from build123d import *

# Parameters (mm, degrees)
SKETCH1_R           = 5
BOSS_EXTRUDE1_DEPTH = 2
BOSS_EXTRUDE2_DEPTH = 65.921828
FILLET1_R           = 12
FILLET2_R           = 12


with BuildPart() as part:
    # Sketch1 → Boss-Extrude1 (new body, symmetric)
    with BuildSketch(Plane(origin=(0, 0, 0), x_dir=(1, 0, 0), z_dir=(0, 1, 0))):
        with BuildLine():
            Line((0, 18), (18, 0))
            Line((18, 0), (96, 0))
            ThreePointArc((96, 0), (104.485281374, 3.514718626), (108, 12))
            Line((108, 12), (108, 26.188792937))
            Line((108, 26.188792937), (54, 64))
            Line((54, 64), (12, 64))
            ThreePointArc((12, 64), (3.514718626, 60.485281374), (0, 52))
            Line((0, 52), (0, 18))
        make_face()
        with Locations((12, 52)):
            Circle(SKETCH1_R, mode=Mode.SUBTRACT)
        with Locations((96, 12)):
            Circle(SKETCH1_R, mode=Mode.SUBTRACT)
    extrude(amount=BOSS_EXTRUDE1_DEPTH, both=True)

    # Sketch4 → Boss-Extrude2 (add)
    with BuildSketch(Plane(origin=(60.164380005, 0, 42.127552411), x_dir=(0.573576436, 0, -0.819152044), z_dir=(0.819152044, 0, 0.573576436))):
        Polygon((83.398858397, 2), (88.643350705, 14.980573964), (92.352086124, 13.48214759), (86.096892465, -2), (83.398858397, -2), align=None)
    extrude(amount=-BOSS_EXTRUDE2_DEPTH)

    # Fillet1
    fillet1_edges = [part.edges().sort_by_distance(p)[0] for p in [
        (82.547528681, -2, -47.30449665),
    ]]
    fillet(fillet1_edges, radius=FILLET1_R)

    # Fillet2
    fillet2_edges = [part.edges().sort_by_distance(p)[0] for p in [
        (81, 2, -45.094396468),
    ]]
    fillet(fillet2_edges, radius=FILLET2_R)


solid = part.part
Here's how the part is built. I have some questions about the finished solid (model axes, mm). A direction names the side the tool comes from. Coordinates: 2 decimals unless noted, no trailing zeros. Loops run counter-clockwise (first coordinate to the right, second up) from the corner with the lowest first, then second, coordinate; pieces in that order, holes last.
1. Imagine slicing it at C-C, the plane y = 4. Please give me the cut outline in (x, z), and give its area (3 significant figures).
2. For faces 5 (the flat face through (52, -2, -27)), 6 (the flat face through (33, 0, -64)), 7 (the flat face through (108, 1, -19)), which set-ups out of +Z, -Z, +X, -X, +Y, -Y let a thin tool reach every point of the face, with its end or its side?
3. If we mould it in two halves opening along X, with no side actions, what happens to faces 1 (the cylindrical face through (100.77, -0.03, -13.5)), 2 (the flat face through (83.743, 12.204, -48.207)), 3 (the cylindrical face through (15, 0, -56)), 4 (the flat face through (41, 2, -25))? For each: pulls with the +X half, pulls with the -X half, needs draft (parallel to the pull), parting line crosses it, or undercut.
4. Imagine slicing it at A-A, the plane z = -13.5. Please give me the cut outline in (x, y).
5. I need wall thicknesses on L1, parallel to X at y = 0.9, z = -52; L2, parallel to Y at x = 72.5, z = -24.5; L3, parallel to X at y = -0.1, z = -12. Which ranges of each line are inside material? Lowest first, please.
6. For P1, Ø3, axis at x = 21.5, z = -26.5, coming from the +Y side; P2, Ø1, axis at x = 94.5, y = 12.5, coming from the +Z side; P3, Ø19, axis at x = 80.5, z = -33.5, coming from the +Y side, each with a flat end and sliding along its axis, tell me the tip position at first contact or that it passes through.
7. Imagine slicing it at B-B, the plane x = 21. Please give me the cut outline in (y, z).
Taken from the geometry:
1. outline: (51.45, -64) - (54, -64) - (56.87, -68.09) - (110.87, -30.28) - (108, -26.19) - (108, -24.41) - close
1. area: 428 mm2
2. face 5: +Z, -Z, +X, -X, -Y
2. face 6: -Z, -X, +Y, -Y
2. face 7: +Z, +X, +Y, -Y
3. face 1: undercut
3. face 2: pulls with the -X half
3. face 3: undercut
3. face 4: needs draft
4. outline: (4.5, -2) - (91.23, -2) - (91.23, 2) - (4.5, 2) - close; (100.77, -2) - (108, -2) - (108, 2) - (100.77, 2) - close
5. L1: x = 0 to 7, 17 to 75.37
5. L2: y = -2 to 2
5. L3: x = 6 to 91, 101 to 108
6. P1: stops at y = 2
6. P2: stops at z = -40.39
6. P3: stops at y = 4.89
7. outline: (-2, -64) - (2, -64) - (2, 0) - (-2, 0) - close
